```python
from build123d import *

# Parameters (mm, degrees)
SKETCH_R        = 2.8
PAD_DEPTH       = 12
SKETCH001_R     = 3.3
POCKET_DEPTH    = 12.001
POCKET001_DEPTH = 6
FILLET_R        = 4
SKETCH003_W     = 13
SKETCH003_H     = 70
POCKET002_DEPTH = 5


with BuildPart() as part:
    # Sketch → Pad (new body)
    with BuildSketch(Plane.XY):
        Polygon((50, 0), (50, 38), (37, 54), (13, 54), (0, 38), (0, 0), (13, -16), (37, -16), align=None)
        with Locations((5, 31)):
            Circle(SKETCH_R, mode=Mode.SUBTRACT)
        with Locations((45, 31)):
            Circle(SKETCH_R, mode=Mode.SUBTRACT)
        with Locations((45, 7)):
            Circle(SKETCH_R, mode=Mode.SUBTRACT)
        with Locations((5, 7)):
            Circle(SKETCH_R, mode=Mode.SUBTRACT)
    extrude(amount=PAD_DEPTH)

    # Sketch001 (on Face14 of Pad) → Pocket (cut, through all)
    with BuildSketch(Plane.XY.offset(12)):
        with Locations((25, 47)):
            Circle(SKETCH001_R)
        with Locations((25, -9)):
            Circle(SKETCH001_R)
    extrude(amount=-POCKET_DEPTH, mode=Mode.SUBTRACT)

    # Sketch002 (on Face4 of Pocket) → Pocket001 (cut)
    with BuildSketch(Plane(origin=(0, 0, 0), x_dir=(1, 0, 0), z_dir=(0, 0, -1))):
        Polygon((27.973354, -52.15), (30.946708, -47), (27.973354, -41.85), (22.026646, -41.85), (19.053292, -47), (22.026646, -52.15), align=None)
        Polygon((27.973354, 3.85), (30.946708, 9), (27.973354, 14.15), (22.026646, 14.15), (19.053292, 9), (22.026646, 3.85), align=None)
    extrude(amount=-POCKET001_DEPTH, mode=Mode.SUBTRACT)

    # Fillet
    fillet_edges = [part.edges().sort_by_distance(p)[0] for p in [
        (0, 38, 6),
        (13, 54, 6),
        (37, 54, 6),
        (0, 0, 6),
        (13, -16, 6),
        (37, -16, 6),
        (50, 0, 6),
        (50, 38, 6),
    ]]
    fillet(fillet_edges, radius=FILLET_R)

    # Sketch003 (on Face5 of Fillet) → Pocket002 (cut)
    with BuildSketch(Plane.XY.offset(12)):
        with Locations((43.5, 19)):
            Rectangle(SKETCH003_W, SKETCH003_H)
    extrude(amount=-POCKET002_DEPTH, mode=Mode.SUBTRACT)


solid = part.part
```
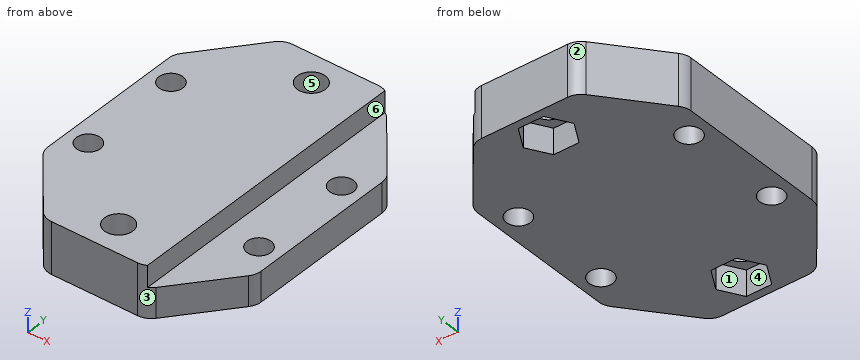
Geometry: final body of the model. Coordinates: model frame, mm. Face numbers are marked on the shaded views. A direction names the side the tool comes from. Round coordinates to 2 decimals unless told otherwise and drop trailing zeros. Order: outer loops, then holes, each group sorted by start corner. A loop starts at its lowest first (then second) coordinate and runs counter-clockwise, first axis right, second up. Notation, with made-up numbers: (2.5, 86) -> (29.5, 86) arc R29 ccw to (29.5, 125) -> close; hole circle Ø2 at (38, 73.25). An arc over 180 degrees is marked (long way). Use one line per item in the form item = value.
(1) Section B-B on x = 25. Return loops of the section in (y, z).
Results list:
outline = (-16, 0) -> (-14.15, 0) -> (-14.15, 6) -> (-12.3, 6) -> (-12.3, 12) -> (-16, 12) -> close; (-5.7, 6) -> (-3.85, 6) -> (-3.85, 0) -> (41.85, 0) -> (41.85, 6) -> (43.7, 6) -> (43.7, 12) -> (-5.7, 12) -> close; (50.3, 6) -> (52.15, 6) -> (52.15, 0) -> (54, 0) -> (54, 12) -> (50.3, 12) -> close
(2) Ray query, probe 1 along Y at (x, z) = (24, 2.25); probe 2 along Y at (x, z) = (45, 4.25); probe 3 along Z at (x, y) = (41, 30.5). Return the intervals inside material, ascending. Write a range as [from, to].
Results list:
probe_1 = [-16, -14.15], [-3.85, 41.85], [52.15, 54]
probe_2 = [-6.15, 4.2], [9.8, 28.2], [33.8, 44.15]
probe_3 = [0, 7]
(3) Section C-C on y = 32. Return loops of the section in (x, z), and give its area (3 significant figures).
Results list:
outline = (0, 0) -> (2.38, 0) -> (2.38, 12) -> (0, 12) -> close; (7.62, 0) -> (42.38, 0) -> (42.38, 7) -> (37, 7) -> (37, 12) -> (7.62, 12) -> close; (47.62, 0) -> (50, 0) -> (50, 7) -> (47.62, 7) -> close
area = 436 mm^2
(4) Draft query along Y for the marked faces 1, 2 and 3. Return one class per face: pulls with the +Y half, pulls with the -Y half, needs draft (parallel to the pull), parting line crosses it, or undercut.
Results list:
face_1 = undercut
face_2 = pulls with the +Y half
face_3 = pulls with the -Y half
(5) Access query for the marked faces 4, 5 and 6. Directions: +Z, -Z, +X, -X, +Y, -Y. A direction counts if a zero-diameter tool reaches every point of the face in a straight line with its end or side. Return the directions, or none.
Results list:
face_4 = -Z
face_5 = +Z, -Z
face_6 = +Z, +X, +Y, -Y
(6) First-contact query: pin 1 Ø14.5 at (x, y) = (46.5, 30.5) entering from +Z; pin 2 Ø3 at (y, z) = (-2, 9) entering from +X; pin 3 Ø1.5 at (x, z) = (6, 2.5) entering from +Y. Flat tips, straight axial feed; report the tip coordinate or a pass-through.
Results list:
pin_1 = 7
pin_2 = 37
pin_3 = 46.31
(7) Section A-A on z = 9. Return loops of the section in (x, y), and give its area (3 significant figures).
Results list:
outline = (0, 1.42) arc R4 ccw to (0.9, -1.1) -> (11.8, -14.52) arc R4 ccw to (14.9, -16) -> (35.1, -16) arc R4 ccw to (37, -15.52) -> (37, 53.52) arc R4 ccw to (35.1, 54) -> (14.9, 54) arc R4 ccw to (11.8, 52.52) -> (0.9, 39.1) arc R4 ccw to (0, 36.58) -> close; hole circle Ø5.6 at (5, 7); hole circle Ø5.6 at (5, 31); hole circle Ø6.6 at (25, -9); hole circle Ø6.6 at (25, 47)
area = 2,260 mm^2
(8) Section D-D on z = 1.25. Count the separate pieces of the cut face and the enclosed holes in it, and give its area (3 significant figures).
Results list:
separate_pieces = 1
enclosed_holes = 6
area = 2,800 mm^2
